The figure shows three views and two pictorial views of one solid part (mm, origin at its lowest corner). Answer the questions. A direction names the side the tool comes from. Round coordinates to 2 decimals unless told otherwise and drop trailing zeros. Order: outer loops, then holes, each group sorted by start corner. A loop starts at its lowest first (then second) coordinate and runs counter-clockwise, first axis right, second up. Notation, with made-up numbers: (16, 82) - (63, 82) arc R25 cw to (63, 104) - close; hole circle Ø10 at (-21, 27.5). An arc over 180 degrees is marked (long way). One line per item, written item: value. Start each with the question number.
1. Section D-D, the plane y = 27.94 is taken. Give the vertices of the cut face in (x, z) (3 decimals).
2. Section A-A, the plane x = 38.1 is taken. Give the vertices of the cut face in (y, z) (3 decimals).
3. Section B-B, the plane x = 25.4 is taken. Give the vertices of the cut face in (y, z) (3 decimals).
4. For a pull along Y with two mould halves and no side action, classify the marked faces 1, 2 and 3 as released by +Y, released by -Y, zero draft, split by the parting line, or undercut.
5. Flat-ended cylindrical pins translate along their axes: P1, Ø3, axis at x = 17, y = 8.5, coming from the +Z side (3 decimals); P2, Ø10, axis at x = 40.5, y = 18, coming from the -Z side; P3, Ø8, axis at x = 17.5, y = 8, coming from the +Z side (3 decimals); P4, Ø6, axis at x = 12.7, z = 79.375, coming from the +Y side. Find the tip coordinate at first contact, or state that the pin passes through.
6. Straight lines are drawn through the part: line 1 (Y direction, x = 12.5, z = 73); line 2 (Z direction, x = 25, y = 14.5) (3 decimals); line 3 (Z direction, x = 12, y = 5) (3 decimals). For each, find the intervals that lie inside material, in ascending order.
7. A tool of negligible diameter and unlimited length cuts with its end or side. For the marked faces 4 and 5, from which of +Z, -Z, +X, -X, +Y, -Y can it reach the whole face along a straight path? Write none if from no direction.
8. Section C-C, the plane y = 11.5 is taken. Give the vertices of the cut face in (x, z) (3 decimals).
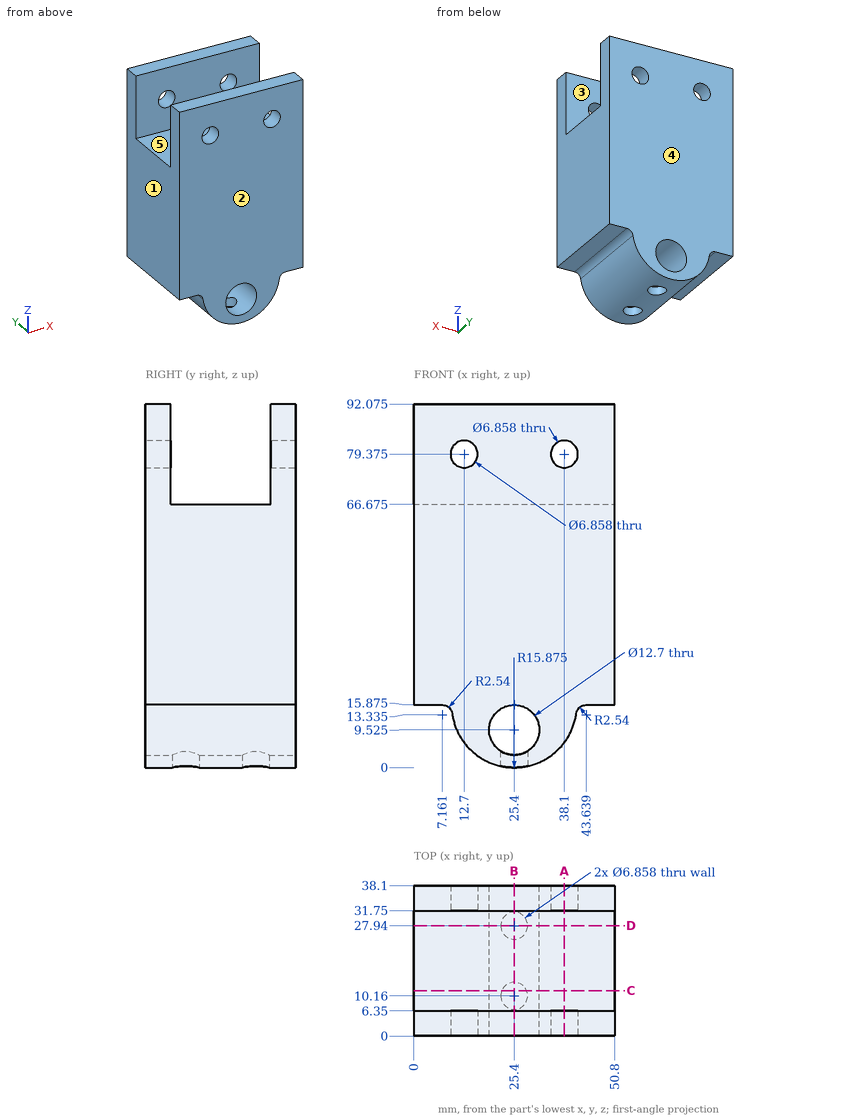
Answer list:
1. outline: (0, 15.875) - (7.161, 15.875) arc R2.54 cw to (9.677, 13.685) arc R15.875 ccw to (21.971, 0.375) - (21.971, 4.18) arc R6.35 cw (long way) to (28.829, 4.18) - (28.829, 0.375) arc R15.875 ccw to (41.123, 13.685) arc R2.54 cw to (43.639, 15.875) - (50.8, 15.875) - (50.8, 66.675) - (0, 66.675) - close
2. outline: (0, 6.35) - (38.1, 6.35) - (38.1, 75.946) - (31.75, 75.946) - (31.75, 66.675) - (6.35, 66.675) - (6.35, 75.946) - (0, 75.946) - close; (0, 82.804) - (6.35, 82.804) - (6.35, 92.075) - (0, 92.075) - close; (31.75, 82.804) - (38.1, 82.804) - (38.1, 92.075) - (31.75, 92.075) - close
3. outline: (0, 0) - (6.731, 0) - (6.731, 3.175) - (0, 3.175) - close; (0, 15.875) - (38.1, 15.875) - (38.1, 92.075) - (31.75, 92.075) - (31.75, 66.675) - (6.35, 66.675) - (6.35, 92.075) - (0, 92.075) - close; (13.589, 0) - (24.511, 0) - (24.511, 3.175) - (13.589, 3.175) - close; (31.369, 0) - (38.1, 0) - (38.1, 3.175) - (31.369, 3.175) - close
4. face 1: zero draft
4. face 2: released by -Y
4. face 3: undercut
5. P1: stops at z = 66.675
5. P2: stops at z = 3.63
5. P3: stops at z = 92.075
5. P4: passes through
6. line 1: y = 0 to 6.35, 31.75 to 38.1
6. line 2: z = 0.005 to 3.188, 15.862 to 66.675
6. line 3: z = 7.363 to 76.018, 82.732 to 92.075
7. face 4: +Z, -Z, +X, -X, +Y
7. face 5: +Z, +X, -X
8. outline: (0, 15.875) - (7.161, 15.875) arc R2.54 cw to (9.677, 13.685) arc R15.875 ccw to (22.244, 0.317) - (22.244, 4.015) arc R6.35 cw (long way) to (28.556, 4.015) - (28.556, 0.317) arc R15.875 ccw to (41.123, 13.685) arc R2.54 cw to (43.639, 15.875) - (50.8, 15.875) - (50.8, 66.675) - (0, 66.675) - close
